Could you check a few things on this model? Use its own coordinates, in mm. Face numbers are marked on the shaded views. A direction names the side the tool comes from. Round coordinates to 2 decimals unless told otherwise and drop trailing zeros. Order: outer loops, then holes, each group sorted by start corner. A loop starts at its lowest first (then second) coordinate and runs counter-clockwise, first axis right, second up. Notation, with made-up numbers: (-14, -6.5) - (13, -6.5) arc R34 cw to (13, 23.5) - close; hole circle Ø9 at (-39, -33). An arc over 180 degrees is marked (long way). Use one line per item in the form item = value.
from build123d import *

# Parameters (mm, degrees)
ESQUISSE1_W                  = 36
ESQUISSE1_H                  = 24
BOSS_EXTRU_1_DEPTH           = 4
ESQUISSE2_R                  = 2
ENL_V_MAT_EXTRU_1_DEPTH      = 1
ENL_V_MAT_EXTRU_1_DEPTH_BACK = 5
BOSS_EXTRU_2_DEPTH           = 36
ESQUISSE4_R                  = 1.65
ENL_V_MAT_EXTRU_2_DEPTH      = 26.11473671
ENL_V_MAT_EXTRU_2_DEPTH_BACK = 10.330127019
CONG_2_R                     = 5
CONG_3_R                     = 2


with BuildPart() as part:
    # Esquisse1 → Boss.-Extru.1 (new body)
    with BuildSketch(Plane.XY):
        with Locations((18, 12)):
            Rectangle(ESQUISSE1_W, ESQUISSE1_H)
    extrude(amount=BOSS_EXTRU_1_DEPTH)

    # Esquisse2 → Enlèv. mat.-Extru.1 (cut, two sides)
    with BuildSketch(Plane.XY.offset(4)) as enl_v_mat_extru_1_sk:
        with Locations((5.5, 10)):
            Circle(ESQUISSE2_R)
        with Locations((30.5, 10)):
            Circle(ESQUISSE2_R)
        with Locations((29.648145657, 16.470476128)):
            Circle(ESQUISSE2_R)
        with Locations((6.351854343, 16.470476128)):
            Circle(ESQUISSE2_R)
    extrude(amount=ENL_V_MAT_EXTRU_1_DEPTH, mode=Mode.SUBTRACT)
    extrude(enl_v_mat_extru_1_sk.sketch, amount=-ENL_V_MAT_EXTRU_1_DEPTH_BACK, mode=Mode.SUBTRACT)

    # Esquisse3 → Boss.-Extru.2 (add)
    with BuildSketch(Plane(origin=(36, 0, 0), x_dir=(0, 0, -1), z_dir=(1, 0, 0))):
        Polygon((0, 24), (8.660254038, 29), (6.660254038, 32.464101615), (-4, 26.309401077), (-4, 24), align=None)
    extrude(amount=-BOSS_EXTRU_2_DEPTH)

    # Esquisse4 → Enlèv. mat.-Extru.2 (cut, two sides)
    with BuildSketch(Plane(origin=(0, 18, 10.392304845), x_dir=(1, 0, 0), z_dir=(0, -0.866025404, -0.5))) as enl_v_mat_extru_2_sk:
        with Locations((8, -17)):
            Circle(ESQUISSE4_R)
        with Locations((28, -17)):
            Circle(ESQUISSE4_R)
    extrude(amount=ENL_V_MAT_EXTRU_2_DEPTH, mode=Mode.SUBTRACT)
    extrude(enl_v_mat_extru_2_sk.sketch, amount=-ENL_V_MAT_EXTRU_2_DEPTH_BACK, mode=Mode.SUBTRACT)

    # Congé2
    cong_2_edges = [part.edges().sort_by_distance(p)[0] for p in [
        (0, 30.732050808, -7.660254038),
        (36, 30.732050808, -7.660254038),
        (36, 0, 2),
        (0, 0, 2),
    ]]
    fillet(cong_2_edges, radius=CONG_2_R)

    # Congé3
    cong_3_edges = [part.edges().sort_by_distance(p)[0] for p in [
        (18, 26.309401077, 4),
        (18, 24, 0),
    ]]
    fillet(cong_3_edges, radius=CONG_3_R)


solid = part.part
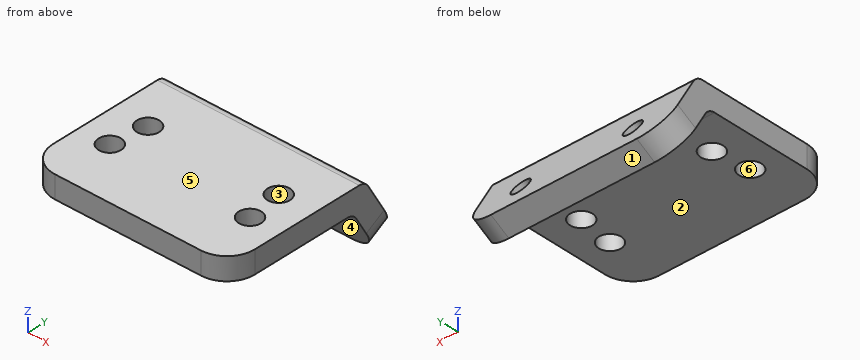
Item 1: Imagine slicing it at A-A on y = 10. Please give me the cut outline in (x, z), plus the area to 3 significant figures.
Found:
outline = (0, 0) - (3.5, 0) - (3.5, 4) - (0, 4) - close; (7.5, 0) - (28.5, 0) - (28.5, 4) - (7.5, 4) - close; (32.5, 0) - (36, 0) - (36, 4) - (32.5, 4) - close
area = 112 mm2
Item 2: Imagine slicing it at C-C on z = 1.5. Please give me the cut outline in (x, y), plus the area to 3 significant figures.
Found:
outline = (0, 5) arc R5 ccw to (5, 0) - (31, 0) arc R5 ccw to (36, 5) - (36, 27.75) - (0, 27.75) - close; hole circle Ø4 at (5.5, 10); hole circle Ø4 at (6.35, 16.47); hole circle Ø4 at (29.65, 16.47); hole circle Ø4 at (30.5, 10)
area = 938 mm2
Item 3: Will these pins go through, and if not, where does the flat tip stop? P1, Ø6.5, axis at x = 29.65, y = 16.47, coming from the -Z side; P2, Ø1.5, axis at x = 31, z = -1, coming from the -Y side; P3, Ø2, axis at x = 5.5, z = -4.5, coming from the -Y side.
Found:
P1 = 0
P2 = 23.81
P3 = 26.02
Item 4: For the marked faces 1 and 2, which set-ups out of +Z, -Z, +X, -X, +Y, -Y let a thin tool reach every point of the face, with its end or its side?
Found:
face_1 = -Z, +X, -X, +Y
face_2 = -Z, +X, -X, -Y
Item 5: Imagine slicing it at D-D on x = 9. Please give me the cut outline in (y, z).
Found:
outline = (0, 0) - (22.85, 0) arc R2 cw to (24.58, -1) - (25.84, -3.19) - (29.31, -1.19) - (26.89, 3) arc R2 ccw to (25.15, 4) - (0, 4) - close; (27.16, -5.47) - (29, -8.66) - (32.46, -6.66) - (30.62, -3.47) - close
Item 6: If we mould it in two halves opening along Y, with no side actions, what happens to the marked faces 3, 4, 5 and 6? For each: released by +Y, released by -Y, zero draft, split by the parting line, or undercut.
Found:
face_3 = undercut
face_4 = released by -Y
face_5 = zero draft
face_6 = undercut
Item 7: I need wall thicknesses on L1, parallel to Y at x = 5.5, z = 1.2; L2, parallel to Z at x = 7, y = 20.5; L3, parallel to Y at x = 18, z = 3. Which ranges of each line are inside material? Lowest first, please.
Found:
L1 = 0 to 8, 12 to 14.66, 18.28 to 27.93
L2 = 0 to 4
L3 = 0 to 26.89
Item 8: Imagine slicing it at B-B on x = 18. Please give me the cut outline in (y, z), plus the area to 3 significant figures.
Found:
outline = (0, 0) - (22.85, 0) arc R2 cw to (24.58, -1) - (29, -8.66) - (32.46, -6.66) - (26.89, 3) arc R2 ccw to (25.15, 4) - (0, 4) - close
area = 145 mm2
